For this review, use the dimensioned drawing (mm, ordinates from the lowest corner) and the shaded views. Give positions to 0.01 mm unless a question says otherwise; leave off trailing zeros. Loops run counter-clockwise (first coordinate to the right, second up) from the corner with the lowest first, then second, coordinate; pieces in that order, holes last. Notation, with made-up numbers: (-33, -15) - (0, -15) arc R27 cw to (0, 1) - close; hole circle Ø6 at (79.25, 35.5). An arc over 180 degrees is marked (long way). Put each result on its own line as item: value.
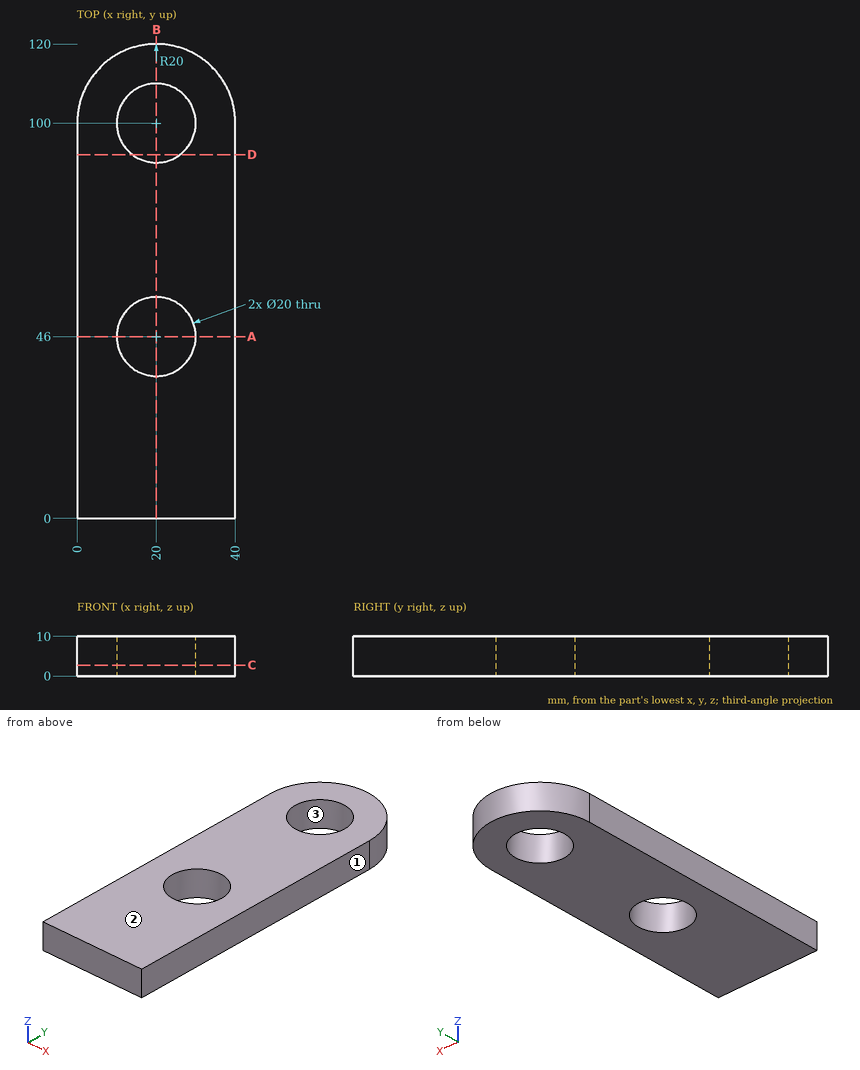
1) Take a section at C-C on z = 2.75. State the section outline as (x, y) points.
Geometry check:
outline: (0, 0) - (40, 0) - (40, 100) arc R20 ccw to (0, 100) - close; hole circle Ø20 at (20, 46); hole circle Ø20 at (20, 100)
2) Take a section at B-B on x = 20. State the section outline as (y, z) points, and give its area (3 significant figures).
Geometry check:
outline: (0, 0) - (36, 0) - (36, 10) - (0, 10) - close; (56, 0) - (90, 0) - (90, 10) - (56, 10) - close; (110, 0) - (120, 0) - (120, 10) - (110, 10) - close
area: 800 mm²
3) Take a section at A-A on y = 46. State the section outline as (x, z) points.
Geometry check:
outline: (0, 0) - (10, 0) - (10, 10) - (0, 10) - close; (30, 0) - (40, 0) - (40, 10) - (30, 10) - close
4) Draft analysis for pull direction X (two halves, no side actions). For the marked faces 1, 2 and 3, state which applies: pulls with the +X half, pulls with the -X half, needs draft (parallel to the pull), parting line crosses it, or undercut.
Geometry check:
face 1: pulls with the +X half
face 2: needs draft
face 3: undercut
5) Take a section at D-D on y = 92. State the section outline as (x, z) points, and give its area (3 significant figures).
Geometry check:
outline: (0, 0) - (14, 0) - (14, 10) - (0, 10) - close; (26, 0) - (40, 0) - (40, 10) - (26, 10) - close
area: 280 mm²
6) Wall thickness on line 1 (Y direction, x = 20, z = 3.25); line 2 (Y direction, x = 17, z = 2.25); line 3 (X direction, y = 93, z = 3.75): over which ranges is each line inside the solid? List them lowest first.
Geometry check:
line 1: y = 0 to 36, 56 to 90, 110 to 120
line 2: y = 0 to 36.46, 55.54 to 90.46, 109.54 to 119.77
line 3: x = 0 to 12.86, 27.14 to 40
7) Insertion check: pin 1 Ø3 at (y, z) = (104.5, 2) entering from +X; pin 2 Ø5 at (x, z) = (27, 6.5) entering from +Y; pin 3 Ø2 at (x, z) = (6, 8.5) entering from -Y; pin 4 Ø1.5 at (x, z) = (26, 7) entering from +Y. Each pin has a flat end and moves straight along its axis. Give the tip position at first contact, or say it passes through.
Geometry check:
pin 1: stops at x = 39.77
pin 2: stops at y = 119.49
pin 3: stops at y = 0
pin 4: stops at y = 119.3
